from build123d import *

# Parameters (mm, degrees)
F0_W     = 5
F0_H     = 2.5
F1_DEPTH = 50
F2_R     = 1.75
F3_DEPTH = 25


with BuildPart() as f1:
    # F0 (on Front) → F1 (new body)
    with BuildSketch(Plane.XZ):
        with Locations((2.5, -1.25)):
            Rectangle(F0_W, F0_H)
    extrude(amount=F1_DEPTH)

    # F2 (on face) → F3 (cut)
    with BuildSketch(Plane.XY):
        with Locations((2.5, -45.636852)):
            Circle(F2_R)
    extrude(amount=-F3_DEPTH, mode=Mode.SUBTRACT)


solid = f1.part
Model file for the job. Use its own axes, mm. Give positions to 0.01 mm unless a question says otherwise; leave off trailing zeros. Order: outer loops, then holes, each group sorted by start corner. A loop starts at its lowest first (then second) coordinate and runs counter-clockwise, first axis right, second up. Notation, with made-up numbers: (50, 48.5) - (97, 48.5) arc R22 cw to (97, 72.5) - close; hole circle Ø9 at (-37.75, 76). An arc over 180 degrees is marked (long way). Return JSON: item names as keys, results as strings.
1) Cut at B-B, the plane z = -1.6. Give the cut face in (x, y).
Geometry says:
{"outline": "(0, -50) - (5, -50) - (5, 0) - (0, 0) - close; hole circle Ø3.5 at (2.5, -45.64)"}
2) Flat gauge pins, fed straight in: P1, Ø1, axis at y = -12.5, z = -1, coming from the -X side; P2, Ø3, axis at x = 2.5, y = -45.64, coming from the +Z side. Where does each tip first touch, or does it go through?
Geometry says:
{"P1": "x = 0", "P2": "through"}
3) Probe line 1 (Y direction, x = 2.5, z = -0.6); line 2 (Y direction, x = 3.55, z = -0.95). List the from-to ranges inside material, lowest first. Write a range as from..to.
Geometry says:
{"line 1": "-50..-47.39, -43.89..0", "line 2": "-50..-47.04, -44.24..0"}
4) Pull direction X, two halves, no side cores. Call faces 1 (the flat face through (0, -25, -1)), 2 (the cylindrical face through (2.121, -47.345, -1.232)), 3 (the flat face through (2, -50, -1)): pulls with the +X half, pulls with the -X half, needs draft (parallel to the pull), parting line crosses it, or undercut.
Geometry says:
{"face 1": "pulls with the -X half", "face 2": "undercut", "face 3": "needs draft"}
5) Cut at A-A, the plane x = 2.5. Give the cut face in (y, z).
Geometry says:
{"outline": "(-50, -2.5) - (-47.39, -2.5) - (-47.39, 0) - (-50, 0) - close; (-43.89, -2.5) - (0, -2.5) - (0, 0) - (-43.89, 0) - close"}
